Could you check a few things on this model? Use its own coordinates, in mm. A direction names the side the tool comes from. Give positions to 0.01 mm unless a question says otherwise; leave off trailing zeros. Order: outer loops, then holes, each group sorted by start corner. A loop starts at its lowest first (then second) coordinate and runs counter-clockwise, first axis right, second up. Notation, with made-up numbers: (11.5, 58.25) - (16.5, 58.25) arc R13 ccw to (16.5, 80.25) - close; hole circle Ø2 at (38.5, 86.25). An arc over 180 degrees is marked (long way). One line per question, with ' | ' between items. Start each with the question number.
1. Imagine slicing it at B-B (x = 7). Please give me the cut outline in (y, z) (3 decimals).
2. For P1, Ø1.6, axis at x = 5, y = 1.5, coming from the +Z side, with a flat end and sliding along its axis, tell me the tip position at first contact or that it passes through.
3. Imagine slicing it at A-A (y = 0.8). Please give me the cut outline in (x, z) (3 decimals).
4. Which directions (+Z, -Z, +X, -X, +Y, -Y) give clear straight access to the entire face, cutting with the end or side of a thin tool? Please do faces 1 (the flat face through (60.401, 2, 10)), 2 (the flat face through (9.601, 2, 10)), 3 (the flat face through (0, 2, -42)).
5. I need wall thicknesses on probe 1 along X at (y, z) = (0.55, 10); probe 2 along Z at (x, y) = (3.5, 2.7); probe 3 along X at (y, z) = (1.1, -41.5). Which ranges of each line are inside material? Lowest first, please. Write a range as from..to.
6. Imagine slicing it at C-C (z = 12.5). Please give me the cut outline in (x, y) (3 decimals).
```python
from build123d import *

# Parameters (mm, degrees)
SKETCH1_W           = 50.8
SKETCH1_H           = 19.4056
BOSS_EXTRUDE1_DEPTH = 3.175


with BuildPart() as part:
    # Sketch1 → Boss-Extrude1 (new body)
    with BuildSketch(Plane(origin=(0, 0, 0), x_dir=(1, 0, 0), z_dir=(0, 1, 0))):
        with Locations((35.0012, -9.7028)):
            Rectangle(SKETCH1_W, SKETCH1_H)
        Polygon((70.0024, 0), (0, 0), (0, 84.9884), (40.005, 84.9884), align=None)
    extrude(amount=BOSS_EXTRUDE1_DEPTH)


solid = part.part
```
Results found:
1) outline: (0, -84.988) - (3.175, -84.988) - (3.175, 0) - (0, 0) - close
2) P1: stops at z = 0
3) outline: (0, -84.988) - (40.005, -84.988) - (70.002, 0) - (60.401, 0) - (60.401, 19.406) - (9.601, 19.406) - (9.601, 0) - (0, 0) - close
4) face 1: +Z, +X, +Y, -Y | face 2: +Z, -X, +Y, -Y | face 3: +Z, -Z, -X, +Y, -Y
5) probe 1: x = 9.6..60.4 | probe 2: z = -84.99..0 | probe 3: x = 0..55.35
6) outline: (9.601, 0) - (60.401, 0) - (60.401, 3.175) - (9.601, 3.175) - close
